Work out the finished part from the listing and answer in its coordinate system (mm). A direction names the side the tool comes from. Round coordinates to 2 decimals unless told otherwise and drop trailing zeros. Loops run counter-clockwise (first coordinate to the right, second up) from the corner with the lowest first, then second, coordinate; pieces in that order, holes last. Notation, with made-up numbers: (64, -5.5) - (85, -5.5) arc R20 cw to (85, 4.5) - close; hole circle Ø3 at (53.25, 56.25). An arc over 180 degrees is marked (long way). Return JSON: item names as keys, results as strings.
from build123d import *

# Parameters (mm, degrees)
SKIZZE1_W                                            = 25
SKIZZE1_H                                            = 23
AUFSATZ_LINEAR_AUSTRAGEN1_DEPTH                      = 6
SKIZZE1_3_W                                          = 17.5
SKIZZE1_3_H                                          = 12.5
SCHNITT_LINEAR_AUSTRAGEN1_DEPTH                      = 5
SKIZZE2_W                                            = 3.75
SKIZZE2_H                                            = 10
SCHNITT_LINEAR_AUSTRAGEN2_DEPTH                      = 5
FORMSENKUNG_F_R_M3_SENKSCHRAUBE_MIT_INNE_D           = 1.6
FORMSENKUNG_F_R_M3_SENKSCHRAUBE_MIT_INNE_CSINK_D     = 3.5
FORMSENKUNG_F_R_M3_SENKSCHRAUBE_MIT_INNE_CSINK_ANGLE = 90
VERRUNDUNG1_R                                        = 2.5


with BuildPart() as part:
    # Skizze1 → Aufsatz-Linear austragen1 (new body)
    with BuildSketch(Plane.XY):
        Rectangle(SKIZZE1_W, SKIZZE1_H)
    extrude(amount=-AUFSATZ_LINEAR_AUSTRAGEN1_DEPTH)

    # Skizze1<3> → Schnitt-Linear austragen1 (cut)
    with BuildSketch(Plane.XY):
        Rectangle(SKIZZE1_3_W, SKIZZE1_3_H)
    extrude(amount=-SCHNITT_LINEAR_AUSTRAGEN1_DEPTH, mode=Mode.SUBTRACT)

    # Skizze2 → Schnitt-Linear austragen2 (cut)
    with BuildSketch(Plane.XY):
        with Locations((-10.625, 0)):
            Rectangle(SKIZZE2_W, SKIZZE2_H)
    extrude(amount=-SCHNITT_LINEAR_AUSTRAGEN2_DEPTH, mode=Mode.SUBTRACT)

    # Formsenkung für M3 Senkschraube mit Innensechskant1 (through all)
    with Locations(Plane(origin=(0, 0, -6), x_dir=(-1, 0, 0), z_dir=(0, 0, -1))):
        with Locations((-10, 9), (10, 9), (10, -9), (-10, -9)):
            CounterSinkHole(FORMSENKUNG_F_R_M3_SENKSCHRAUBE_MIT_INNE_D / 2, FORMSENKUNG_F_R_M3_SENKSCHRAUBE_MIT_INNE_CSINK_D / 2, counter_sink_angle=FORMSENKUNG_F_R_M3_SENKSCHRAUBE_MIT_INNE_CSINK_ANGLE)

    # Verrundung1
    verrundung1_edges = [part.edges().sort_by_distance(p)[0] for p in [
        (-12.5, 11.5, -3),
        (12.5, 11.5, -3),
        (12.5, -11.5, -3),
        (-12.5, -11.5, -3),
    ]]
    fillet(verrundung1_edges, radius=VERRUNDUNG1_R)


solid = part.part
1) A tool of negligible diameter and unlimited length cuts with its end or side. For faces 1 (the cylindrical face through (11.748, -10.787, -3.042)), 2 (the flat face through (0, 6.25, -2)), from which of +Z, -Z, +X, -X, +Y, -Y can it reach the whole face along a straight path? Write none if from no direction.
Verdict:
{"face 1": "+Z, -Z, +X, -Y", "face 2": "+Z"}
2) Find the intervals of material crossed by L1, parallel to X at y = 9, z = -2.25; L2, parallel to Y at x = 10, z = -2; L3, parallel to Y at x = -4, z = -0.85, in increasing order.
Verdict:
{"L1": "x = -12.5 to -10.8, -9.2 to 9.2, 10.8 to 12.5", "L2": "y = -11.5 to -9.8, -8.2 to 8.2, 9.8 to 11.5", "L3": "y = -11.5 to -6.25, 6.25 to 11.5"}
3) Flat-ended cylindrical pins translate along their axes: pin 1 (2.5 mm diameter, centred on y = -1, z = -1.5, fed in from -X); pin 2 (2 mm diameter, centred on x = 10, y = -9, fed in from -Z); pin 3 (2 mm diameter, centred on x = 5, y = -3.5, fed in from +Z). Find the tip coordinate at first contact, or state that the pin passes through.
Verdict:
{"pin 1": "stops at x = 8.75", "pin 2": "stops at z = -5.25", "pin 3": "stops at z = -5"}
4) Determine the mould class of faces 3 (the flat face through (0, 0, -6)), 4 (the flat face through (-8.75, 6, -2)), 5 (the cylindrical face through (11.787, 10.748, -3.042)) for opening direction Y: pulls with the +Y half, pulls with the -Y half, needs draft (parallel to the pull), parting line crosses it, or undercut.
Verdict:
{"face 3": "needs draft", "face 4": "undercut", "face 5": "pulls with the +Y half"}
5) Section A-A (z = -4.65) is taken. Give the vertices of the cut face in (x, y).
Verdict:
{"outline": "(-12.5, -9) arc R2.5 ccw to (-10, -11.5) - (10, -11.5) arc R2.5 ccw to (12.5, -9) - (12.5, 9) arc R2.5 ccw to (10, 11.5) - (-10, 11.5) arc R2.5 ccw to (-12.5, 9) - (-12.5, 5) - (-8.75, 5) - (-8.75, 6.25) - (8.75, 6.25) - (8.75, -6.25) - (-8.75, -6.25) - (-8.75, -5) - (-12.5, -5) - close; hole circle Ø1.6 at (-10, -9); hole circle Ø1.6 at (-10, 9); hole circle Ø1.6 at (10, -9); hole circle Ø1.6 at (10, 9)"}
6) Section B-B (y = 3.5) is taken. Give the vertices of the cut face in (x, z), and give its area (4 significant figures).
Verdict:
{"outline": "(-12.5, -6) - (12.5, -6) - (12.5, 0) - (8.75, 0) - (8.75, -5) - (-12.5, -5) - close", "area": "43.75 mm2"}
